```python
from build123d import *

# Parameters (mm, degrees)
SKETCH1_R                      = 44.45
SKETCH1_R_2                    = 3.25
BOSS_EXTRUDE1_DEPTH            = 3.175
BOSS_EXTRUDE2_DEPTH            = 25.4
CBORE_FOR_M6_SHCS2_D           = 7
CBORE_FOR_M6_SHCS2_CBORE_D     = 11
CBORE_FOR_M6_SHCS2_CBORE_DEPTH = 6
SKETCH10_W                     = 206.275362682
SKETCH10_H                     = 234.398565581
CUT_EXTRUDE1_DEPTH             = 15.2875
CBORE_FOR_M6_SHCS3_D           = 7
CBORE_FOR_M6_SHCS3_CBORE_D     = 11
CBORE_FOR_M6_SHCS3_CBORE_DEPTH = 8.54


with BuildPart() as part:
    # Sketch1 → Boss-Extrude1 (new body)
    with BuildSketch(Plane(origin=(0, 0, 0), x_dir=(1, 0, 0), z_dir=(0, 1, 0))):
        with BuildLine():
            Line((-57.15, 63.5), (57.15, 63.5))
            ThreePointArc((57.15, 63.5), (61.640128061, 61.640128061), (63.5, 57.15))
            Line((63.5, 57.15), (63.5, -57.15))
            ThreePointArc((63.5, -57.15), (61.640128061, -61.640128061), (57.15, -63.5))
            Line((57.15, -63.5), (-57.15, -63.5))
            ThreePointArc((-57.15, -63.5), (-61.640128061, -61.640128061), (-63.5, -57.15))
            Line((-63.5, -57.15), (-63.5, 57.15))
            ThreePointArc((-63.5, 57.15), (-61.640128061, 61.640128061), (-57.15, 63.5))
        make_face()
        Circle(SKETCH1_R, mode=Mode.SUBTRACT)
        with Locations((-57.15, 53.975)):
            Circle(SKETCH1_R_2, mode=Mode.SUBTRACT)
        with Locations((57.15, 53.975)):
            Circle(SKETCH1_R_2, mode=Mode.SUBTRACT)
        with Locations((57.15, -53.975)):
            Circle(SKETCH1_R_2, mode=Mode.SUBTRACT)
        with Locations((-57.15, -53.975)):
            Circle(SKETCH1_R_2, mode=Mode.SUBTRACT)
    extrude(amount=BOSS_EXTRUDE1_DEPTH)

    # Sketch3 → Boss-Extrude2 (add)
    with BuildSketch(Plane(origin=(0, 3.175, 0), x_dir=(1, 0, 0), z_dir=(0, 1, 0))):
        with BuildLine():
            Line((-57.15, -63.5), (57.15, -63.5))
            ThreePointArc((57.15, -63.5), (61.640128061, -61.640128061), (63.5, -57.15))
            Line((63.5, -57.15), (63.5, 57.15))
            ThreePointArc((63.5, 57.15), (61.640128061, 61.640128061), (57.15, 63.5))
            Line((57.15, 63.5), (-57.15, 63.5))
            ThreePointArc((-57.15, 63.5), (-61.640128061, 61.640128061), (-63.5, 57.15))
            Line((-63.5, 57.15), (-63.5, -57.15))
            ThreePointArc((-63.5, -57.15), (-61.640128061, -61.640128061), (-57.15, -63.5))
        make_face()
        with BuildLine():
            Line((-54.700256121, 45.358975516), (-45.358975516, 54.700256121))
            ThreePointArc((-45.358975516, 54.700256121), (-41.238798986, 57.453270063), (-36.378719395, 58.42))
            Line((-36.378719395, 58.42), (36.378719395, 58.42))
            ThreePointArc((36.378719395, 58.42), (41.238798986, 57.453270063), (45.358975516, 54.700256121))
            Line((45.358975516, 54.700256121), (54.700256121, 45.358975516))
            ThreePointArc((54.700256121, 45.358975516), (57.453270063, 41.238798986), (58.42, 36.378719395))
            Line((58.42, 36.378719395), (58.42, -36.378719395))
            ThreePointArc((58.42, -36.378719395), (57.453270063, -41.238798986), (54.700256121, -45.358975516))
            Line((54.700256121, -45.358975516), (45.358975516, -54.700256121))
            ThreePointArc((45.358975516, -54.700256121), (41.238798986, -57.453270063), (36.378719395, -58.42))
            Line((36.378719395, -58.42), (-36.378719395, -58.42))
            ThreePointArc((-36.378719395, -58.42), (-41.238798986, -57.453270063), (-45.358975516, -54.700256121))
            Line((-45.358975516, -54.700256121), (-54.700256121, -45.358975516))
            ThreePointArc((-54.700256121, -45.358975516), (-57.453270063, -41.238798986), (-58.42, -36.378719395))
            Line((-58.42, -36.378719395), (-58.42, 36.378719395))
            ThreePointArc((-58.42, 36.378719395), (-57.453270063, 41.238798986), (-54.700256121, 45.358975516))
        make_face(mode=Mode.SUBTRACT)
    extrude(amount=BOSS_EXTRUDE2_DEPTH)

    # CBORE for M6 SHCS2 (through all)
    with Locations(Plane(origin=(0, 0, 0), x_dir=(-1, 0, 0), z_dir=(0, -1, 0))):
        with Locations((-55.88, 55.88), (55.88, 55.88), (55.88, -55.88), (-55.88, -55.88)):
            CounterBoreHole(CBORE_FOR_M6_SHCS2_D / 2, CBORE_FOR_M6_SHCS2_CBORE_D / 2, CBORE_FOR_M6_SHCS2_CBORE_DEPTH)

    # Sketch10 → Cut-Extrude1 (cut, through all)
    with BuildSketch(Plane(origin=(0, 14.2875, 0), x_dir=(-1, 0, 0), z_dir=(0, -1, 0))):
        with Locations((4.587579463, 2.84706708)):
            Rectangle(SKETCH10_W, SKETCH10_H)
    extrude(amount=CUT_EXTRUDE1_DEPTH, mode=Mode.SUBTRACT)

    # CBORE for M6 SHCS3 (through all)
    with Locations(Plane(origin=(0, 28.575, 0), x_dir=(1, 0, 0), z_dir=(0, 1, 0))):
        with Locations((55.88, 55.88), (55.88, -55.88), (-55.88, -55.88), (-55.88, 55.88)):
            CounterBoreHole(CBORE_FOR_M6_SHCS3_D / 2, CBORE_FOR_M6_SHCS3_CBORE_D / 2, CBORE_FOR_M6_SHCS3_CBORE_DEPTH)


solid = part.part
```
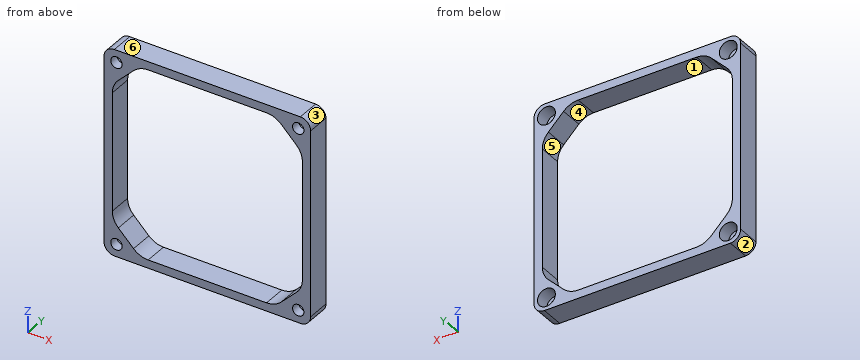
The listing builds one solid part. Answer for the finished solid, in the listing's coordinates (mm). Face numbers are marked on the shaded views. A direction names the side the tool comes from. Give positions to 0.01 mm unless a question says otherwise; leave off trailing zeros. Loops run counter-clockwise (first coordinate to the right, second up) from the corner with the lowest first, then second, coordinate; pieces in that order, holes last. Notation, with made-up numbers: (71.5, 63) - (129.5, 63) arc R14 ccw to (129.5, 69) - close; hole circle Ø7 at (45, -34). An arc over 180 degrees is marked (long way). Answer as CSV lines item,"result". Start each with the question number.
Item 1: Find the intervals of material crossed by line 1 (Z direction, x = 14, y = 26); line 2 (X direction, y = 26.25, z = 55.88), in increasing order. Write a range as from..to.
Item 2: A cutting plane is placed at B-B on z = -34. Determine the outline of the cut face in (x, y) (1 decimal).
Item 3: A cutting plane is placed at C-C on y = 25.5. Determine the outline of the cut face in (x, z), then the cut area to 3 significant figures.
Item 4: Each of these flat-tipped pins is pushed along its axis until it touches: pin 1 (12 mm diameter, centred on x = 55.5, z = 57.5, fed in from +Y) (3 decimals); pin 2 (3.5 mm diameter, centred on x = -58, z = -53.5, fed in from +Y) (3 decimals). Where does it stop, or does it pass through?
Item 5: For the marked faces 1 and 2, determine the directions among +Z, -Z, +X, -X, +Y, -Y from which every point of the face is accessible in a straight line to the end or side of a thin tool.
Item 6: The mould has two halves that part along X. Classify the marked faces 3, 4, 5 and 6: +X half, -X half, draft (parallel to the pull), parting line (faces both ways), or undercut.
Item 7: A cutting plane is placed at A-A on x = -31. Determine the outline of the cut face in (y, z) (1 decimal).
Found:
1,line 1,"z = -63.5..-58.42, 58.42..63.5"
1,line 2,"x = -63.5..-61.38, -50.38..-44, 44..50.38, 61.38..63.5"
2,outline,"(-63.5, 14.3) - (-58.4, 14.3) - (-58.4, 28.6) - (-63.5, 28.6) - close; (58.4, 14.3) - (63.5, 14.3) - (63.5, 28.6) - (58.4, 28.6) - close"
3,outline,"(-63.5, -57.15) arc R6.35 ccw to (-57.15, -63.5) - (57.15, -63.5) arc R6.35 ccw to (63.5, -57.15) - (63.5, 57.15) arc R6.35 ccw to (57.15, 63.5) - (-57.15, 63.5) arc R6.35 ccw to (-63.5, 57.15) - close; hole circle Ø11 at (-55.88, -55.88); hole circle Ø11 at (-55.88, 55.88); hole (-58.42, -36.38) arc R12.7 ccw to (-54.7, -45.36) - (-45.36, -54.7) arc R12.7 ccw to (-36.38, -58.42) - (36.38, -58.42) arc R12.7 ccw to (45.36, -54.7) - (54.7, -45.36) arc R12.7 ccw to (58.42, -36.38) - (58.42, 36.38) arc R12.7 ccw to (54.7, 45.36) - (45.36, 54.7) arc R12.7 ccw to (36.38, 58.42) - (-36.38, 58.42) arc R12.7 ccw to (-45.36, 54.7) - (-54.7, 45.36) arc R12.7 ccw to (-58.42, 36.38) - close; hole circle Ø11 at (55.88, -55.88); hole circle Ø11 at (55.88, 55.88)"
3,area,"2,650 mm^2"
4,pin 1,"stops at y = 28.575"
4,pin 2,"stops at y = 20.035"
5,face 1,"+Y, -Y"
5,face 2,"-Z, -X, +Y, -Y"
6,face 3,"+X half"
6,face 4,"undercut"
6,face 5,"undercut"
6,face 6,"draft"
7,outline,"(14.3, -63.5) - (28.6, -63.5) - (28.6, -58.4) - (14.3, -58.4) - close; (14.3, 58.4) - (28.6, 58.4) - (28.6, 63.5) - (14.3, 63.5) - close"
